from build123d import *

# Parameters (mm, degrees)
BOSS_EXTRUDE1_DEPTH = 14
SKETCH2_R           = 2
CUT_EXTRUDE2_DEPTH  = 9


with BuildPart() as part:
    # Sketch1 → Boss-Extrude1 (new body)
    with BuildSketch(Plane.XY):
        with BuildLine():
            ThreePointArc((-0.158092835, 3.754907593), (-0.451477513, 3.047309694), (-1.159482409, 2.754908559))
            ThreePointArc((-1.159482409, 2.754908559), (-3.799725402, 3.002497057), (-6.349938035, 3.729544963))
            ThreePointArc((-6.349938035, 3.729544963), (-7.060326346, 3.93180492), (-7.795792236, 4))
            Line((-7.795792236, 4), (-20, 4))
            ThreePointArc((-20, 4), (-22, 2), (-20, 0))
            Line((-20, 0), (0, 0))
            Line((0, 0), (0, -2))
            Line((0, -2), (-20, -2))
            ThreePointArc((-20, -2), (-24, 2), (-20, 6))
            Line((-20, 6), (-7.410531978, 6))
            ThreePointArc((-7.410531978, 6), (-6.631548949, 5.923415023), (-5.882395119, 5.696592721))
            ThreePointArc((-5.882395119, 5.696592721), (-3.565674535, 4.994277462), (-1.156703262, 4.754906628))
            ThreePointArc((-1.156703262, 4.754906628), (-0.450494936, 4.461522915), (-0.158092835, 3.754907593))
        make_face()
    extrude(amount=BOSS_EXTRUDE1_DEPTH)

    # Sketch2 → Cut-Extrude2 (cut, through all)
    with BuildSketch(Plane(origin=(0, -2, 0), x_dir=(-1, 0, 0), z_dir=(0, -1, 0))):
        with Locations((10, -7)):
            Circle(SKETCH2_R)
    extrude(amount=-CUT_EXTRUDE2_DEPTH, mode=Mode.SUBTRACT)


solid = part.part
Read the model definition and answer for the solid it produces. Units are mm, in the model's axes. A direction names the side the tool comes from. Coordinates: 2 decimals unless noted, no trailing zeros. Loops run counter-clockwise (first coordinate to the right, second up) from the corner with the lowest first, then second, coordinate; pieces in that order, holes last. Notation, with made-up numbers: (4, 20) -> (9, 20) arc R14 cw to (9, 26) -> close; hole circle Ø5 at (31, 24). An arc over 180 degrees is marked (long way). Write item = value, one per line. Start each with the question number.
1) The part is cut by section C-C, the plane z = 7. Determine the outline of the cut face in (x, y), plus the area to 3 significant figures.
2) Find the intervals of material crossed by L1, parallel to Y at x = -18, z = 2.5; L2, parallel to Z at x = -10, y = 5.4; L3, parallel to Y at x = -2, z = 7, in increasing order. Write a range as from..to.
3) The part is cut by section A-A, the plane x = -10. Determine the outline of the cut face in (y, z), plus the area to 3 significant figures.
4) Given P1, Ø1, axis at y = -1, z = 2.5, coming from the -X side; P2, Ø1.5, axis at y = 3, z = 1.5, coming from the +X side; P3, Ø2.5, axis at x = -10, z = 7, coming from the -Y side, each flat-ended and moving along its own axis, determine where each tip first touches the part or whether it passes through.
5) For faces 4 (the face through (-14, 4, 7)), 5 (the face through (-12.4, 0, 6.9)), 6 (the face through (-8.4, 5, 8.2)), determine the directions among +Z, -Z, +X, -X, +Y, -Y from which every point of the face is accessible in a straight line to the end or side of a thin tool.
6) The part is cut by section B-B, the plane x = -17. Determine the outline of the cut face in (y, z), plus the area to 3 significant figures.
7) The mould has two halves that part along Z. Classify faces 1 (the face through (-3.763, 2.996, 6.902)), 2 (the face through (-12, -1, 14)), 3 (the face through (-8.4, -1, 8.2)): pulls with the +Z half, pulls with the -Z half, needs draft (parallel to the pull), parting line crosses it, or undercut.
8) The part is cut by section D-D, the plane z = 11.25. Determine the outline of the cut face in (x, y), plus the area to 3 significant figures.
Result:
q1.outline = (-20, -2) -> (-12, -2) -> (-12, 0) -> (-20, 0) arc R2 cw to (-20, 4) -> (-12, 4) -> (-12, 6) -> (-20, 6) arc R4 ccw to start; (-8, -2) -> (0, -2) -> (0, 0) -> (-8, 0) -> close; (-8, 4) -> (-7.8, 4) arc R4 cw to (-6.35, 3.73) arc R14.41 ccw to (-1.16, 2.75) arc R1 ccw to (-1.16, 4.75) arc R12.41 cw to (-5.88, 5.7) arc R4 ccw to (-7.41, 6) -> (-8, 6) -> close
q1.area = 82.5 mm²
q2.L1 = -2..0, 4..6
q2.L2 = 0..5, 9..14
q2.L3 = -2..0, 2.78..4.78
q3.outline = (-2, 0) -> (0, 0) -> (0, 5) -> (-2, 5) -> close; (-2, 9) -> (0, 9) -> (0, 14) -> (-2, 14) -> close; (4, 0) -> (6, 0) -> (6, 5) -> (4, 5) -> close; (4, 9) -> (6, 9) -> (6, 14) -> (4, 14) -> close
q3.area = 40.0 mm²
q4.P1 = -23.12
q4.P2 = -0.16
q4.P3 = through
q5.face_4 = +Z, -Z
q5.face_5 = +Z, -Z, +X
q5.face_6 = +Y, -Y
q6.outline = (-2, 0) -> (0, 0) -> (0, 14) -> (-2, 14) -> close; (4, 0) -> (6, 0) -> (6, 14) -> (4, 14) -> close
q6.area = 56.0 mm²
q7.face_1 = needs draft
q7.face_2 = pulls with the +Z half
q7.face_3 = undercut
q8.outline = (-20, -2) -> (0, -2) -> (0, 0) -> (-20, 0) arc R2 cw to (-20, 4) -> (-7.8, 4) arc R4 cw to (-6.35, 3.73) arc R14.41 ccw to (-1.16, 2.75) arc R1 ccw to (-1.16, 4.75) arc R12.41 cw to (-5.88, 5.7) arc R4 ccw to (-7.41, 6) -> (-20, 6) arc R4 ccw to start
q8.area = 98.5 mm²
